Here's how the part is built. I have some questions about the finished solid (model axes, mm). A direction names the side the tool comes from. Give positions to 0.01 mm unless a question says otherwise; leave off trailing zeros. Order: outer loops, then holes, each group sorted by start corner. A loop starts at its lowest first (then second) coordinate and runs counter-clockwise, first axis right, second up. Notation, with made-up numbers: (55, 19.25) - (60, 19.25) arc R23 ccw to (60, 47.25) - close; hole circle Ø4 at (65.5, 32.25). An arc over 180 degrees is marked (long way). One line per question, with ' | ' between items.
from build123d import *

# Parameters (mm, degrees)
BOSS_EXTRUDE1_DEPTH = 28
SKETCH2_R           = 1.4
SKETCH2_R_2         = 5.5
CUT_EXTRUDE1_DEPTH  = 69.361978468
CUT_EXTRUDE2_REACH  = 85.714
SKETCH3_R           = 1.5
CUT_EXTRUDE3_REACH  = 85.714
SKETCH4_R           = 1.6
SKETCH6_R           = 2
CUT_EXTRUDE5_DEPTH  = 2
SKETCH7_R           = 2.65
CUT_EXTRUDE6_DEPTH  = 2
FILLET1_R           = 10
FILLET2_R           = 2
BOSS_EXTRUDE2_DEPTH = 12
SKETCH10_W          = 3.9
SKETCH10_H          = 28
BOSS_EXTRUDE3_DEPTH = 12.5
CUT_EXTRUDE8_REACH  = 85.714
SKETCH8_R           = 1.5
CUT_EXTRUDE9_START  = -1.5
SKETCH11_R          = 2.75
SKETCH11_R_2        = 1.5
CUT_EXTRUDE9_DEPTH  = 1.5
FILLET3_R           = 3
FILLET4_R           = 1
SKETCH12_R          = 2.65
SKETCH12_R_2        = 1.5
CUT_EXTRUDE10_DEPTH = 1


with BuildPart() as part:
    # Sketch1 → Boss-Extrude1 (new body)
    with BuildSketch(Plane(origin=(0, 0, 0), x_dir=(1, 0, 0), z_dir=(0, 1, 0))):
        Polygon((-27.62, -36.95), (27.62, -36.95), (27.62, 36.95), (-27.62, 36.95), (-27.62, 32.95), (22.62, 32.95), (22.62, -32.95), (-27.62, -32.95), align=None)
    extrude(amount=BOSS_EXTRUDE1_DEPTH)

    # Sketch2 → Cut-Extrude1 (cut, through all)
    with BuildSketch(Plane.ZY.offset(-22.62)):
        with Locations((0, 4)):
            Circle(SKETCH2_R)
        with Locations((0, 24)):
            Circle(SKETCH2_R)
        with Locations((-10, 14)):
            Circle(SKETCH2_R)
        with Locations((10, 14)):
            Circle(SKETCH2_R)
        with Locations((0, 14)):
            Circle(SKETCH2_R_2)
    extrude(amount=-CUT_EXTRUDE1_DEPTH, mode=Mode.SUBTRACT)

    # Sketch3 → Cut-Extrude2 (cut, up to next)
    with BuildSketch(Plane.XY.offset(36.95), mode=Mode.PRIVATE) as cut_extrude2_sk1:
        with Locations((1.62, 14)):
            Circle(SKETCH3_R)
    cut_extrude2_tool1 = extrude(cut_extrude2_sk1.sketch, amount=-CUT_EXTRUDE2_REACH, mode=Mode.PRIVATE) & part.part
    add(cut_extrude2_tool1.solids().sort_by_distance((1.62, 14, 36.95))[0], mode=Mode.SUBTRACT)

    # Sketch4 → Cut-Extrude3 (cut, up to next)
    with BuildSketch(Plane(origin=(0, 0, -36.95), x_dir=(-1, 0, 0), z_dir=(0, 0, -1)), mode=Mode.PRIVATE) as cut_extrude3_sk1:
        with Locations((-1.62, 14)):
            Circle(SKETCH4_R)
    cut_extrude3_tool1 = extrude(cut_extrude3_sk1.sketch, amount=-CUT_EXTRUDE3_REACH, mode=Mode.PRIVATE) & part.part
    add(cut_extrude3_tool1.solids().sort_by_distance((1.62, 14, -36.95))[0], mode=Mode.SUBTRACT)

    # Sketch6 → Cut-Extrude5 (cut)
    with BuildSketch(Plane(origin=(27.62, 0, 0), x_dir=(0, 0, -1), z_dir=(1, 0, 0))):
        with Locations((0, 24)):
            Circle(SKETCH6_R)
        with Locations((10, 14)):
            Circle(SKETCH6_R)
        with Locations((0, 4)):
            Circle(SKETCH6_R)
        with Locations((-10, 14)):
            Circle(SKETCH6_R)
    extrude(amount=-CUT_EXTRUDE5_DEPTH, mode=Mode.SUBTRACT)

    # Sketch7 → Cut-Extrude6 (cut)
    with BuildSketch(Plane(origin=(0, 0, -36.95), x_dir=(-1, 0, 0), z_dir=(0, 0, -1))):
        with Locations((-1.62, 14)):
            Circle(SKETCH7_R)
    extrude(amount=-CUT_EXTRUDE6_DEPTH, mode=Mode.SUBTRACT)

    # Fillet1
    fillet1_edges = [part.edges().sort_by_distance(p)[0] for p in [
        (-27.62, 0, 34.95),
        (-27.62, 28, 34.95),
        (-27.62, 28, -34.95),
        (-27.62, 0, -34.95),
    ]]
    fillet(fillet1_edges, radius=FILLET1_R)

    # Fillet2
    fillet2_edges = [part.edges().sort_by_distance(p)[0] for p in [
        (27.62, 14, -36.95),
        (27.62, 14, 36.95),
        (22.62, 14, 32.95),
        (22.62, 14, -32.95),
    ]]
    fillet(fillet2_edges, radius=FILLET2_R)

    # Sketch9 → Boss-Extrude2 (add)
    with BuildSketch(Plane(origin=(0, 0, 32.95), x_dir=(-1, 0, 0), z_dir=(0, 0, -1))):
        with BuildLine():
            Line((17.62, 28), (17.62, 0))
            ThreePointArc((17.62, 0), (24.691067812, 2.928932188), (27.62, 10))
            Line((27.62, 10), (27.62, 18))
            ThreePointArc((27.62, 18), (24.691067812, 25.071067812), (17.62, 28))
        make_face()
    extrude(amount=BOSS_EXTRUDE2_DEPTH)

    # Sketch10 → Boss-Extrude3 (add)
    with BuildSketch(Plane(origin=(-17.62, 0, 0), x_dir=(0, 0, -1), z_dir=(1, 0, 0))):
        with Locations((-22.9, 14)):
            Rectangle(SKETCH10_W, SKETCH10_H)
    extrude(amount=BOSS_EXTRUDE3_DEPTH)

    # Cut-Extrude8: up to this face of the body (flat: up to its plane)
    cut_extrude8_end = Plane(part.part.faces().sort_by_distance((-15.710832536, 14, 20.95))[0])
    # Sketch8 → Cut-Extrude8 (cut, up to the picked face)
    with BuildSketch(Plane.XY.offset(36.95), mode=Mode.PRIVATE) as cut_extrude8_sk1:
        with Locations(Location((-8.13, 14, 0), (0, 0, 90))):
            Circle(SKETCH8_R)
    cut_extrude8_tool1 = split(extrude(cut_extrude8_sk1.sketch, amount=-CUT_EXTRUDE8_REACH, mode=Mode.PRIVATE), bisect_by=cut_extrude8_end, keep=Keep.BOTH, mode=Mode.PRIVATE)
    add(cut_extrude8_tool1.solids().sort_by(Axis((-8.13, 14, 36.95), (0, 0, -1)))[0], mode=Mode.SUBTRACT)

    # Sketch11 → Cut-Extrude9 (cut)
    with BuildSketch(Plane(origin=(0, 0, 20.95), x_dir=(-1, 0, 0), z_dir=(0, 0, -1)).offset(CUT_EXTRUDE9_START)):
        with Locations((8.13, 14)):
            Circle(SKETCH11_R)
        with Locations(Location((8.13, 14, 0), (0, 0, 90))):
            Circle(SKETCH11_R_2, mode=Mode.SUBTRACT)
    extrude(amount=CUT_EXTRUDE9_DEPTH, mode=Mode.SUBTRACT)

    # Fillet3
    fillet3_edges = [part.edges().sort_by_distance(p)[0] for p in [
        (-5.12, 0, 22.9),
        (-5.12, 28, 22.9),
    ]]
    fillet(fillet3_edges, radius=FILLET3_R)

    # Fillet4
    fillet4_edges = [part.edges().sort_by_distance(p)[0] for p in [
        (-17.62, 14, 32.95),
        (-17.62, 14, 24.85),
    ]]
    fillet(fillet4_edges, radius=FILLET4_R)

    # Sketch12 → Cut-Extrude10 (cut)
    with BuildSketch(Plane.XY.offset(36.95)):
        with Locations(Location((1.62, 14, 0), (0, 0, 180))):
            Circle(SKETCH12_R)
        with Locations((1.62, 14)):
            Circle(SKETCH12_R_2, mode=Mode.SUBTRACT)
    extrude(amount=-CUT_EXTRUDE10_DEPTH, mode=Mode.SUBTRACT)


solid = part.part
1) I'm going to push flat-ended pins straight in: P1, Ø3.5, axis at y = 14, z = -10, coming from the -X side; P2, Ø5, axis at x = 1.62, y = 14, coming from the -Z side; P3, Ø3.5, axis at y = 24, z = 0, coming from the +X side; P4, Ø2, axis at y = 14, z = -10, coming from the -X side. Where does each tip first touch, or does it pass through?
Model answer:
P1: stops at x = 22.62 | P2: stops at z = -34.95 | P3: stops at x = 25.62 | P4: passes through
2) I want a section at C-C (z = 0). List the corners of the cut face in (x, y) for me, plus the area to 3 significant figures.
Model answer:
outline: (22.62, 0) - (27.62, 0) - (27.62, 2) - (25.62, 2) - (25.62, 2.6) - (22.62, 2.6) - close; (22.62, 5.4) - (25.62, 5.4) - (25.62, 6) - (27.62, 6) - (27.62, 8.5) - (22.62, 8.5) - close; (22.62, 19.5) - (27.62, 19.5) - (27.62, 22) - (25.62, 22) - (25.62, 22.6) - (22.62, 22.6) - close; (22.62, 25.4) - (25.62, 25.4) - (25.62, 26) - (27.62, 26) - (27.62, 28) - (22.62, 28) - close | area: 52.2 mm2
3) Please list where these lines run through material, in increasing order: L1, parallel to Z at x = -6, y = 23.5; L2, parallel to Y at x = 27, z = 0; L3, parallel to Y at x = 1.62, z = 35.2.
Model answer:
L1: z = -36.95 to -32.95, 20.95 to 24.85, 32.95 to 36.95 | L2: y = 0 to 2, 6 to 8.5, 19.5 to 22, 26 to 28 | L3: y = 0 to 12.5, 15.5 to 28
4) On a 3-axis mill with a long thin cutter (end or side, diameter ignored), from which of +Z, -Z, +X, -X, +Y, -Y can I reach the whole of each face in a straight line? I mean faces 5 (the face through (-5.98, 27.1, 22.87)), 6 (the face through (22.05, 14.2, -32.35)), 7 (the face through (-9.3, 12.8, 22.45)), 8 (the face through (-17.62, 14, 29)). Say none if no direction works.
Model answer:
face 5: +Y | face 6: -X, +Y, -Y | face 7: none | face 8: +Y, -Y
5) I want a section at D-D (x = 1.62). List the corners of the cut face in (y, z) for me.
Model answer:
outline: (0, -36.95) - (11.35, -36.95) - (11.35, -34.95) - (12.4, -34.95) - (12.4, -32.95) - (0, -32.95) - close; (0, 32.95) - (12.5, 32.95) - (12.5, 35.95) - (11.35, 35.95) - (11.35, 36.95) - (0, 36.95) - close; (15.5, 32.95) - (28, 32.95) - (28, 36.95) - (16.65, 36.95) - (16.65, 35.95) - (15.5, 35.95) - close; (15.6, -34.95) - (16.65, -34.95) - (16.65, -36.95) - (28, -36.95) - (28, -32.95) - (15.6, -32.95) - close
6) Thinking about a two-plate mould opening in Z: for faces 1 (the face through (0, 15, 35.95)), 2 (the face through (0.397, 16.351, 36.457)), 3 (the face through (24.099, 2.633, -0.303)), 4 (the face through (27.05, 14.2, -36.35)), which applies, +Z half, -Z half, draft (parallel to the pull), parting line (faces both ways), or undercut?
Model answer:
face 1: +Z half | face 2: draft | face 3: undercut | face 4: -Z half
7) I want a section at A-A (z = -10). List the corners of the cut face in (x, y) for me, plus the area to 3 significant figures.
Model answer:
outline: (22.62, 0) - (27.62, 0) - (27.62, 12) - (25.62, 12) - (25.62, 12.6) - (22.62, 12.6) - close; (22.62, 15.4) - (25.62, 15.4) - (25.62, 16) - (27.62, 16) - (27.62, 28) - (22.62, 28) - close | area: 124 mm2
8) I want a section at B-B (x = 24). List the corners of the cut face in (y, z) for me.
Model answer:
outline: (0, -36.95) - (28, -36.95) - (28, 36.95) - (0, 36.95) - close; hole circle Ø2.8 at (4, 0); hole circle Ø11 at (14, 0); hole circle Ø2.8 at (14, -10); hole circle Ø2.8 at (14, 10); hole circle Ø2.8 at (24, 0)
